The model under review builds one solid part; all positions refer to its coordinate system, in mm. Round coordinates to 2 decimals unless told otherwise and drop trailing zeros. Write each loop counter-clockwise with the first axis right and the second up, starting at its lowest first coordinate (ties: lowest second). Pieces come first, ordered by that corner, then holes. Notation, with made-up numbers: (7, -6.75) -> (57, -6.75) arc R34 cw to (57, 24.25) -> close; hole circle Ø10 at (-3.5, -38.5). An arc over 180 degrees is marked (long way). Answer in a Markdown table with one row per item. Add a question column.
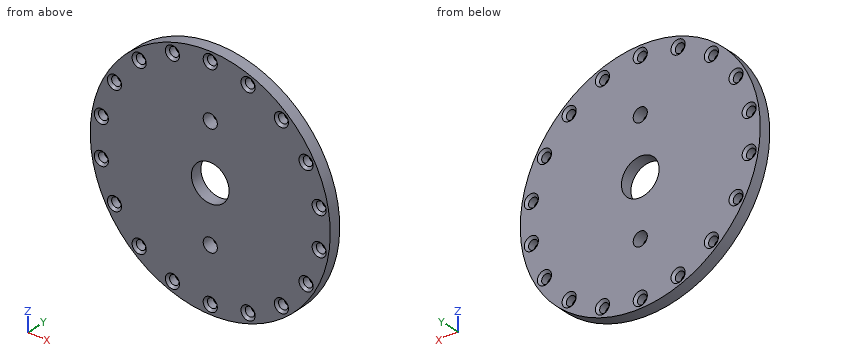
```python
from build123d import *

# Parameters (mm, degrees)
SKETCH1_R           = 25.5
BOSS_EXTRUDE1_DEPTH = 2.5
CUT_EXTRUDE1_REACH  = 38.149
SKETCH2_R           = 4
CUT_EXTRUDE2_REACH  = 38.149
SKETCH3_R           = 1.5
CUT_EXTRUDE3_REACH  = 38.149
SKETCH4_R           = 1
CHAMFER1_SIZE       = 0.5


with BuildPart() as part:
    # Sketch1 → Boss-Extrude1 (new body)
    with BuildSketch(Plane(origin=(0, 0, 0), x_dir=(1, 0, 0), z_dir=(0, 1, 0))):
        with Locations(Location((0, 0, 0), (0, 0, 270))):
            Circle(SKETCH1_R)
    extrude(amount=BOSS_EXTRUDE1_DEPTH)

    # Sketch2 → Cut-Extrude1 (cut, up to next)
    with BuildSketch(Plane(origin=(0, 0, 0), x_dir=(1, 0, 0), z_dir=(0, 1, 0)), mode=Mode.PRIVATE) as cut_extrude1_sk1:
        with Locations(Location((0, 0, 0), (0, 0, 270))):
            Circle(SKETCH2_R)
    cut_extrude1_tool1 = extrude(cut_extrude1_sk1.sketch, amount=CUT_EXTRUDE1_REACH, mode=Mode.PRIVATE) & part.part
    add(cut_extrude1_tool1.solids().sort_by_distance((0, 0, 0))[0], mode=Mode.SUBTRACT)

    # Sketch3 → Cut-Extrude2 (cut, up to next)
    with BuildSketch(Plane(origin=(0, 0, 0), x_dir=(1, 0, 0), z_dir=(0, 1, 0)), mode=Mode.PRIVATE) as cut_extrude2_sk1:
        with Locations(Location((0, 12, 0), (0, 0, 270))):
            Circle(SKETCH3_R)
    cut_extrude2_tool1 = extrude(cut_extrude2_sk1.sketch, amount=CUT_EXTRUDE2_REACH, mode=Mode.PRIVATE) & part.part
    # Sketch3 → Cut-Extrude2 (cut, up to next)
    with BuildSketch(Plane(origin=(0, 0, 0), x_dir=(1, 0, 0), z_dir=(0, 1, 0)), mode=Mode.PRIVATE) as cut_extrude2_sk2:
        with Locations(Location((0, -12, 0), (0, 0, 270))):
            Circle(SKETCH3_R)
    cut_extrude2_tool2 = extrude(cut_extrude2_sk2.sketch, amount=CUT_EXTRUDE2_REACH, mode=Mode.PRIVATE) & part.part
    add(cut_extrude2_tool1.solids().sort_by_distance((0, 0, -12))[0], mode=Mode.SUBTRACT)
    add(cut_extrude2_tool2.solids().sort_by_distance((0, 0, 12))[0], mode=Mode.SUBTRACT)

    # Sketch4 → Cut-Extrude3 (cut, up to next)
    with BuildSketch(Plane(origin=(0, 0, 0), x_dir=(1, 0, 0), z_dir=(0, 1, 0)), mode=Mode.PRIVATE) as cut_extrude3_sk1:
        with Locations(Location((0, 23.5, 0), (0, 0, 270))):
            Circle(SKETCH4_R)
    cut_extrude3_tool1 = extrude(cut_extrude3_sk1.sketch, amount=CUT_EXTRUDE3_REACH, mode=Mode.PRIVATE) & part.part
    # Sketch4 → Cut-Extrude3 (cut, up to next)
    with BuildSketch(Plane(origin=(0, 0, 0), x_dir=(1, 0, 0), z_dir=(0, 1, 0)), mode=Mode.PRIVATE) as cut_extrude3_sk2:
        with Locations(Location((8.037473368, 22.082776588, 0), (0, 0, 270))):
            Circle(SKETCH4_R)
    cut_extrude3_tool2 = extrude(cut_extrude3_sk2.sketch, amount=CUT_EXTRUDE3_REACH, mode=Mode.PRIVATE) & part.part
    # Sketch4 → Cut-Extrude3 (cut, up to next)
    with BuildSketch(Plane(origin=(0, 0, 0), x_dir=(1, 0, 0), z_dir=(0, 1, 0)), mode=Mode.PRIVATE) as cut_extrude3_sk3:
        with Locations(Location((15.105508828, 18.002044413, 0), (0, 0, 270))):
            Circle(SKETCH4_R)
    cut_extrude3_tool3 = extrude(cut_extrude3_sk3.sketch, amount=CUT_EXTRUDE3_REACH, mode=Mode.PRIVATE) & part.part
    # Sketch4 → Cut-Extrude3 (cut, up to next)
    with BuildSketch(Plane(origin=(0, 0, 0), x_dir=(1, 0, 0), z_dir=(0, 1, 0)), mode=Mode.PRIVATE) as cut_extrude3_sk4:
        with Locations(Location((20.351596989, 11.75, 0), (0, 0, 270))):
            Circle(SKETCH4_R)
    cut_extrude3_tool4 = extrude(cut_extrude3_sk4.sketch, amount=CUT_EXTRUDE3_REACH, mode=Mode.PRIVATE) & part.part
    # Sketch4 → Cut-Extrude3 (cut, up to next)
    with BuildSketch(Plane(origin=(0, 0, 0), x_dir=(1, 0, 0), z_dir=(0, 1, 0)), mode=Mode.PRIVATE) as cut_extrude3_sk5:
        with Locations(Location((23.142982196, 4.080732175, 0), (0, 0, 270))):
            Circle(SKETCH4_R)
    cut_extrude3_tool5 = extrude(cut_extrude3_sk5.sketch, amount=CUT_EXTRUDE3_REACH, mode=Mode.PRIVATE) & part.part
    # Sketch4 → Cut-Extrude3 (cut, up to next)
    with BuildSketch(Plane(origin=(0, 0, 0), x_dir=(1, 0, 0), z_dir=(0, 1, 0)), mode=Mode.PRIVATE) as cut_extrude3_sk6:
        with Locations(Location((23.142982196, -4.080732175, 0), (0, 0, 270))):
            Circle(SKETCH4_R)
    cut_extrude3_tool6 = extrude(cut_extrude3_sk6.sketch, amount=CUT_EXTRUDE3_REACH, mode=Mode.PRIVATE) & part.part
    # Sketch4 → Cut-Extrude3 (cut, up to next)
    with BuildSketch(Plane(origin=(0, 0, 0), x_dir=(1, 0, 0), z_dir=(0, 1, 0)), mode=Mode.PRIVATE) as cut_extrude3_sk7:
        with Locations(Location((20.351596989, -11.75, 0), (0, 0, 270))):
            Circle(SKETCH4_R)
    cut_extrude3_tool7 = extrude(cut_extrude3_sk7.sketch, amount=CUT_EXTRUDE3_REACH, mode=Mode.PRIVATE) & part.part
    # Sketch4 → Cut-Extrude3 (cut, up to next)
    with BuildSketch(Plane(origin=(0, 0, 0), x_dir=(1, 0, 0), z_dir=(0, 1, 0)), mode=Mode.PRIVATE) as cut_extrude3_sk8:
        with Locations(Location((15.105508828, -18.002044413, 0), (0, 0, 270))):
            Circle(SKETCH4_R)
    cut_extrude3_tool8 = extrude(cut_extrude3_sk8.sketch, amount=CUT_EXTRUDE3_REACH, mode=Mode.PRIVATE) & part.part
    # Sketch4 → Cut-Extrude3 (cut, up to next)
    with BuildSketch(Plane(origin=(0, 0, 0), x_dir=(1, 0, 0), z_dir=(0, 1, 0)), mode=Mode.PRIVATE) as cut_extrude3_sk9:
        with Locations(Location((8.037473368, -22.082776588, 0), (0, 0, 270))):
            Circle(SKETCH4_R)
    cut_extrude3_tool9 = extrude(cut_extrude3_sk9.sketch, amount=CUT_EXTRUDE3_REACH, mode=Mode.PRIVATE) & part.part
    # Sketch4 → Cut-Extrude3 (cut, up to next)
    with BuildSketch(Plane(origin=(0, 0, 0), x_dir=(1, 0, 0), z_dir=(0, 1, 0)), mode=Mode.PRIVATE) as cut_extrude3_sk10:
        with Locations(Location((0, -23.5, 0), (0, 0, 270))):
            Circle(SKETCH4_R)
    cut_extrude3_tool10 = extrude(cut_extrude3_sk10.sketch, amount=CUT_EXTRUDE3_REACH, mode=Mode.PRIVATE) & part.part
    # Sketch4 → Cut-Extrude3 (cut, up to next)
    with BuildSketch(Plane(origin=(0, 0, 0), x_dir=(1, 0, 0), z_dir=(0, 1, 0)), mode=Mode.PRIVATE) as cut_extrude3_sk11:
        with Locations(Location((-8.037473368, -22.082776588, 0), (0, 0, 270))):
            Circle(SKETCH4_R)
    cut_extrude3_tool11 = extrude(cut_extrude3_sk11.sketch, amount=CUT_EXTRUDE3_REACH, mode=Mode.PRIVATE) & part.part
    # Sketch4 → Cut-Extrude3 (cut, up to next)
    with BuildSketch(Plane(origin=(0, 0, 0), x_dir=(1, 0, 0), z_dir=(0, 1, 0)), mode=Mode.PRIVATE) as cut_extrude3_sk12:
        with Locations(Location((-15.105508828, -18.002044413, 0), (0, 0, 270))):
            Circle(SKETCH4_R)
    cut_extrude3_tool12 = extrude(cut_extrude3_sk12.sketch, amount=CUT_EXTRUDE3_REACH, mode=Mode.PRIVATE) & part.part
    # Sketch4 → Cut-Extrude3 (cut, up to next)
    with BuildSketch(Plane(origin=(0, 0, 0), x_dir=(1, 0, 0), z_dir=(0, 1, 0)), mode=Mode.PRIVATE) as cut_extrude3_sk13:
        with Locations(Location((-20.351596989, -11.75, 0), (0, 0, 270))):
            Circle(SKETCH4_R)
    cut_extrude3_tool13 = extrude(cut_extrude3_sk13.sketch, amount=CUT_EXTRUDE3_REACH, mode=Mode.PRIVATE) & part.part
    # Sketch4 → Cut-Extrude3 (cut, up to next)
    with BuildSketch(Plane(origin=(0, 0, 0), x_dir=(1, 0, 0), z_dir=(0, 1, 0)), mode=Mode.PRIVATE) as cut_extrude3_sk14:
        with Locations(Location((-23.142982196, -4.080732175, 0), (0, 0, 270))):
            Circle(SKETCH4_R)
    cut_extrude3_tool14 = extrude(cut_extrude3_sk14.sketch, amount=CUT_EXTRUDE3_REACH, mode=Mode.PRIVATE) & part.part
    # Sketch4 → Cut-Extrude3 (cut, up to next)
    with BuildSketch(Plane(origin=(0, 0, 0), x_dir=(1, 0, 0), z_dir=(0, 1, 0)), mode=Mode.PRIVATE) as cut_extrude3_sk15:
        with Locations(Location((-23.142982196, 4.080732175, 0), (0, 0, 270))):
            Circle(SKETCH4_R)
    cut_extrude3_tool15 = extrude(cut_extrude3_sk15.sketch, amount=CUT_EXTRUDE3_REACH, mode=Mode.PRIVATE) & part.part
    # Sketch4 → Cut-Extrude3 (cut, up to next)
    with BuildSketch(Plane(origin=(0, 0, 0), x_dir=(1, 0, 0), z_dir=(0, 1, 0)), mode=Mode.PRIVATE) as cut_extrude3_sk16:
        with Locations(Location((-20.351596989, 11.75, 0), (0, 0, 270))):
            Circle(SKETCH4_R)
    cut_extrude3_tool16 = extrude(cut_extrude3_sk16.sketch, amount=CUT_EXTRUDE3_REACH, mode=Mode.PRIVATE) & part.part
    # Sketch4 → Cut-Extrude3 (cut, up to next)
    with BuildSketch(Plane(origin=(0, 0, 0), x_dir=(1, 0, 0), z_dir=(0, 1, 0)), mode=Mode.PRIVATE) as cut_extrude3_sk17:
        with Locations(Location((-15.105508828, 18.002044413, 0), (0, 0, 270))):
            Circle(SKETCH4_R)
    cut_extrude3_tool17 = extrude(cut_extrude3_sk17.sketch, amount=CUT_EXTRUDE3_REACH, mode=Mode.PRIVATE) & part.part
    # Sketch4 → Cut-Extrude3 (cut, up to next)
    with BuildSketch(Plane(origin=(0, 0, 0), x_dir=(1, 0, 0), z_dir=(0, 1, 0)), mode=Mode.PRIVATE) as cut_extrude3_sk18:
        with Locations(Location((-8.037473368, 22.082776588, 0), (0, 0, 270))):
            Circle(SKETCH4_R)
    cut_extrude3_tool18 = extrude(cut_extrude3_sk18.sketch, amount=CUT_EXTRUDE3_REACH, mode=Mode.PRIVATE) & part.part
    add(cut_extrude3_tool1.solids().sort_by_distance((0, 0, -23.5))[0], mode=Mode.SUBTRACT)
    add(cut_extrude3_tool2.solids().sort_by_distance((8.037473, 0, -22.082777))[0], mode=Mode.SUBTRACT)
    add(cut_extrude3_tool3.solids().sort_by_distance((15.105509, 0, -18.002044))[0], mode=Mode.SUBTRACT)
    add(cut_extrude3_tool4.solids().sort_by_distance((20.351597, 0, -11.75))[0], mode=Mode.SUBTRACT)
    add(cut_extrude3_tool5.solids().sort_by_distance((23.142982, 0, -4.080732))[0], mode=Mode.SUBTRACT)
    add(cut_extrude3_tool6.solids().sort_by_distance((23.142982, 0, 4.080732))[0], mode=Mode.SUBTRACT)
    add(cut_extrude3_tool7.solids().sort_by_distance((20.351597, 0, 11.75))[0], mode=Mode.SUBTRACT)
    add(cut_extrude3_tool8.solids().sort_by_distance((15.105509, 0, 18.002044))[0], mode=Mode.SUBTRACT)
    add(cut_extrude3_tool9.solids().sort_by_distance((8.037473, 0, 22.082777))[0], mode=Mode.SUBTRACT)
    add(cut_extrude3_tool10.solids().sort_by_distance((0, 0, 23.5))[0], mode=Mode.SUBTRACT)
    add(cut_extrude3_tool11.solids().sort_by_distance((-8.037473, 0, 22.082777))[0], mode=Mode.SUBTRACT)
    add(cut_extrude3_tool12.solids().sort_by_distance((-15.105509, 0, 18.002044))[0], mode=Mode.SUBTRACT)
    add(cut_extrude3_tool13.solids().sort_by_distance((-20.351597, 0, 11.75))[0], mode=Mode.SUBTRACT)
    add(cut_extrude3_tool14.solids().sort_by_distance((-23.142982, 0, 4.080732))[0], mode=Mode.SUBTRACT)
    add(cut_extrude3_tool15.solids().sort_by_distance((-23.142982, 0, -4.080732))[0], mode=Mode.SUBTRACT)
    add(cut_extrude3_tool16.solids().sort_by_distance((-20.351597, 0, -11.75))[0], mode=Mode.SUBTRACT)
    add(cut_extrude3_tool17.solids().sort_by_distance((-15.105509, 0, -18.002044))[0], mode=Mode.SUBTRACT)
    add(cut_extrude3_tool18.solids().sort_by_distance((-8.037473, 0, -22.082777))[0], mode=Mode.SUBTRACT)

    # Chamfer1
    chamfer1_edges = [part.edges().sort_by_distance(p)[0] for p in [
        (0, 0, -24.5),
        (0, 2.5, -24.5),
        (8.037473368, 0, -23.082776588),
        (8.037473368, 2.5, -23.082776588),
        (15.105508828, 0, -19.002044413),
        (15.105508828, 2.5, -19.002044413),
        (20.351596989, 0, -12.75),
        (20.351596989, 2.5, -12.75),
        (23.142982196, 0, -5.080732175),
        (23.142982196, 2.5, -5.080732175),
        (23.142982196, 0, 3.080732175),
        (23.142982196, 2.5, 3.080732175),
        (20.351596989, 0, 10.75),
        (20.351596989, 2.5, 10.75),
        (15.105508828, 0, 17.002044413),
        (15.105508828, 2.5, 17.002044413),
        (8.037473368, 0, 21.082776588),
        (8.037473368, 2.5, 21.082776588),
        (0, 0, 22.5),
        (0, 2.5, 22.5),
        (-8.037473368, 0, 21.082776588),
        (-8.037473368, 2.5, 21.082776588),
        (-15.105508828, 0, 17.002044413),
        (-15.105508828, 2.5, 17.002044413),
        (-20.351596989, 0, 10.75),
        (-20.351596989, 2.5, 10.75),
        (-23.142982196, 0, 3.080732175),
        (-23.142982196, 2.5, 3.080732175),
        (-23.142982196, 0, -5.080732175),
        (-23.142982196, 2.5, -5.080732175),
        (-20.351596989, 0, -12.75),
        (-20.351596989, 2.5, -12.75),
        (-15.105508828, 0, -19.002044413),
        (-15.105508828, 2.5, -19.002044413),
        (-8.037473368, 0, -23.082776588),
        (-8.037473368, 2.5, -23.082776588),
    ]]
    chamfer(chamfer1_edges, length=CHAMFER1_SIZE)


solid = part.part
```
1. Add section C-C on z = 11.75. Write out the cut boundary in (x, y), plus the area to 3 significant figures.
2. Add section A-A on x = 0. State how many separate pieces and enclosed holes the cut face has, plus the area to 3 significant figures.
3. Add section B-B on z = 0. Write out the cut boundary in (x, y).
4. Insertion check: pin 1 Ø2.5 at (x, z) = (-20.35, -11.75) entering from +Y; pin 2 Ø2.5 at (x, z) = (-23.14, 4.08) entering from -Y. Each pin has a flat end and moves straight along its axis. Give the tip position at first contact, or say it passes through.
5. For L1, parallel to X at y = 1.9, z = -12; L2, parallel to X at y = 1.15, z = 11.75; L3, parallel to Z at x = 22.5, y = 2.3, list the stretches that pass through material, from the lowest coordinate up.
Filled in:
| question | item | result |
|---|---|---|
| 1 | outline | (-22.63, 0) -> (-21.85, 0) -> (-21.35, 0.5) -> (-21.35, 2) -> (-21.85, 2.5) -> (-22.63, 2.5) -> close; (-19.35, 0.5) -> (-18.85, 0) -> (-1.48, 0) -> (-1.48, 2.5) -> (-18.85, 2.5) -> (-19.35, 2) -> close; (1.48, 0) -> (18.85, 0) -> (19.35, 0.5) -> (19.35, 2) -> (18.85, 2.5) -> (1.48, 2.5) -> close; (21.35, 0.5) -> (21.85, 0) -> (22.63, 0) -> (22.63, 2.5) -> (21.85, 2.5) -> (21.35, 2) -> close |
| 1 | area | 94.8 mm² |
| 2 | separate pieces | 6 |
| 2 | enclosed holes | 0 |
| 2 | area | 81.5 mm² |
| 3 | outline | (-25.5, 0) -> (-4, 0) -> (-4, 2.5) -> (-25.5, 2.5) -> close; (4, 0) -> (25.5, 0) -> (25.5, 2.5) -> (4, 2.5) -> close |
| 4 | pin 1 | y = 2.25 |
| 4 | pin 2 | y = 0.25 |
| 5 | L1 | -22.5 to -21.32, -19.38 to -1.5, 1.5 to 19.38, 21.32 to 22.5 |
| 5 | L2 | -22.63 to -21.35, -19.35 to -1.48, 1.48 to 19.35, 21.35 to 22.63 |
| 5 | L3 | -12 to -5.21, -2.95 to 2.95, 5.21 to 12 |
